from build123d import *

# Parameters (mm, degrees)
SKETCH1_R               = 35
SKETCH1_R_2             = 20
BOSS_EXTRUDE1_DEPTH     = 75
CUT_EXTRUDE1_DEPTH      = 45
CUT_EXTRUDE1_DEPTH_BACK = 54
CUT_EXTRUDE2_DEPTH      = 48
CUT_EXTRUDE2_DEPTH_BACK = 44
CUT_EXTRUDE3_DEPTH      = 44
CUT_EXTRUDE3_DEPTH_BACK = 44
SKETCH4_R               = 7.5


with BuildPart() as part:
    # Sketch1 → Boss-Extrude1 (new body)
    with BuildSketch(Plane.XY):
        Circle(SKETCH1_R)
        Circle(SKETCH1_R_2, mode=Mode.SUBTRACT)
    extrude(amount=BOSS_EXTRUDE1_DEPTH)

    # Sketch2 → Cut-Extrude1 (cut, two sides: drawn at the far end of the back side and taken through both)
    with BuildSketch(Plane(origin=(0, 0, 0), x_dir=(0, 0, -1), z_dir=(1, 0, 0)).offset(-CUT_EXTRUDE1_DEPTH_BACK)):
        with BuildLine():
            Line((0, -35), (0, 0))
            ThreePointArc((0, 0), (-4.127707746, -9.965168023), (-14.092875769, -14.092875769))
            Line((-14.092875769, -14.092875769), (-25.439318665, -14.092875769))
            Line((-25.439318665, -14.092875769), (-52.150222161, -35))
            Line((-52.150222161, -35), (0, -35))
        make_face()
        with BuildLine():
            Line((-25.439318665, 14.092875769), (-14.092875769, 14.092875769))
            ThreePointArc((-14.092875769, 14.092875769), (-4.127707746, 9.965168023), (0, 0))
            Line((0, 0), (0, 35))
            Line((0, 35), (-51.84345844, 35))
            Line((-51.84345844, 35), (-25.439318665, 14.092875769))
        make_face()
    extrude(amount=CUT_EXTRUDE1_DEPTH + CUT_EXTRUDE1_DEPTH_BACK, mode=Mode.SUBTRACT)

    # Sketch3 → Cut-Extrude2 (cut, two sides: drawn at the far end of the back side and taken through both)
    with BuildSketch(Plane(origin=(0, 0, 0), x_dir=(1, 0, 0), z_dir=(0, 1, 0)).offset(-CUT_EXTRUDE2_DEPTH_BACK)):
        with BuildLine():
            Line((-27.558791769, 0), (-27.558791769, -25.439318665))
            ThreePointArc((-27.558791769, -25.439318665), (0.052095226, -46.7551788), (27.662982221, -25.439318665))
            Line((27.662982221, -25.439318665), (27.662982221, 0))
            Line((27.662982221, 0), (-27.558791769, 0))
        make_face()
    extrude(amount=CUT_EXTRUDE2_DEPTH + CUT_EXTRUDE2_DEPTH_BACK, mode=Mode.SUBTRACT)

    # Sketch4 → Cut-Extrude3 (cut, two sides: drawn at the far end of the back side and taken through both)
    with BuildSketch(Plane(origin=(0, 0, 0), x_dir=(0, 0, -1), z_dir=(1, 0, 0)).offset(-CUT_EXTRUDE3_DEPTH_BACK)):
        with Locations(Location((-12.483344887, 0, 0), (0, 0, 180))):
            Circle(SKETCH4_R)
    extrude(amount=CUT_EXTRUDE3_DEPTH + CUT_EXTRUDE3_DEPTH_BACK, mode=Mode.SUBTRACT)


solid = part.part
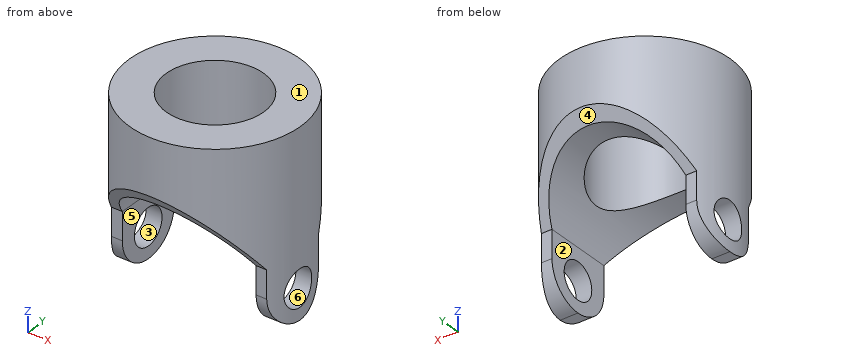
Check sheet for the modelled part. Datum: model origin and axes. Units: mm. Face numbers are marked on the shaded views. A direction names the side the tool comes from. Give positions to 0.01 mm unless a question says otherwise; leave off trailing zeros. Write each loop counter-clockwise with the first axis right and the second up, starting at its lowest first coordinate (ties: lowest second). Pieces come first, ordered by that corner, then holes. Notation, with made-up numbers: (15, 82.5) -> (25, 82.5) arc R29 ccw to (25, 117.5) -> close; hole circle Ø11 at (27.5, 84.25). An arc over 180 degrees is marked (long way). Use one line per item in the form item = value. Start each with the question number.
1. Section check C-C (z = 67). Record the cut outline in (x, y), and give its area (3 significant figures).
2. Mould release check, pull along Z, two halves, no side actions. Record for the marked faces 1, 2, 3 and 4: pulls with the +Z half, pulls with the -Z half, needs draft (parallel to the pull), parting line crosses it, or undercut.
3. Go/stop test with flat-tipped pins: P1, Ø4, axis at y = 17.5, z = 66, coming from the -X side; P2, Ø10, axis at x = 12, z = 60.5, coming from the -Y side; P3, Ø2, axis at x = -29, z = 22.5, coming from the -Y side. Record where each tip stops, or that it passes through.
4. Section check B-B (x = -17.5). Record the cut outline in (y, z), and give its area (3 significant figures).
5. Section check A-A (y = -1). Record the cut outline in (x, z).
6. Section check D-D (z = 27.5). Record the cut outline in (x, y), and give its area (3 significant figures).
7. Access from +Z, -Z, +X, -X, +Y, -Y to the whole of each face (thin tool, end or side, straight path). Record for the marked faces 5 and 6.
8. Thickness scan on line 1 along X through (y, z) = (3, 42.5); line 2 along Z through (x, y) = (-0.5, 26); line 3 along X through (y, z) = (-13.5, 26). Record the ranges inside material, lowest first. Write a range as from..to.
Conclusion:
q1.outline = circle Ø70 at (0, 0); hole circle Ø40 at (0, 0)
q1.area = 2,590 mm²
q2.face_1 = pulls with the +Z half
q2.face_2 = needs draft
q2.face_3 = undercut
q2.face_4 = pulls with the -Z half
q3.P1 = -31.38
q3.P2 = -34.29
q3.P3 = -14.09
q4.outline = (-30.31, 46.16) -> (-26.05, 40.72) -> (-9.68, 40.72) -> (-9.68, 75) -> (-30.31, 75) -> close; (9.68, 40.72) -> (26.19, 40.72) -> (30.31, 45.92) -> (30.31, 75) -> (9.68, 75) -> close
q4.area = 1,390 mm²
q5.outline = (-34.99, 0.04) -> (-27.56, 0.04) -> (-27.56, 5.05) -> (-34.99, 5.05) -> close; (-34.99, 19.92) -> (-27.56, 19.92) -> (-27.56, 25.44) arc R28.54 cw to (-19.97, 38.55) -> (-19.97, 75) -> (-34.99, 75) -> close; (19.97, 38.65) arc R28.54 cw to (27.66, 25.44) -> (27.66, 19.92) -> (34.99, 19.92) -> (34.99, 75) -> (19.97, 75) -> close; (27.66, 0.04) -> (34.99, 0.04) -> (34.99, 5.05) -> (27.66, 5.05) -> close
q6.outline = (-31.28, -15.71) -> (-26.94, -15.71) -> (-26.94, 15.72) -> (-31.27, 15.72) arc R35 ccw to start; (27.04, -15.71) -> (31.28, -15.71) arc R35 ccw to (31.27, 15.72) -> (27.04, 15.72) -> close
q6.area = 427 mm²
q7.face_5 = -Z, +Y, -Y
q7.face_6 = +X, -X
q8.line_1 = -34.87..-19.77, 19.77..34.87
q8.line_2 = 46.75..75
q8.line_3 = -32.29..-27.41, 27.51..32.29
